Can you work these out from the model? Positions are in its coordinate system, mm. Face numbers are marked on the shaded views. A direction names the side the tool comes from. Coordinates: 2 decimals unless noted, no trailing zeros. Write each loop counter-clockwise with the first axis right and the second up, starting at its lowest first coordinate (ties: lowest second). Pieces come first, ordered by that corner, then holes. Notation, with made-up numbers: (39, 14) -> (63, 14) arc R25 cw to (63, 32) -> close; hole circle Ø3 at (84, 14). An arc over 180 degrees is marked (long way). Use one line per item in the form item = value.
```python
from build123d import *

# Parameters (mm, degrees)
F0_W     = 16
F0_H     = 16
F1_DEPTH = 220
F2_R     = 7.99999
F3_R     = 7.5
F4_DEPTH = 20


# Not quite as in the source:
# - a fillet or chamfer is up to 0.001 mm smaller than in the source, because OpenCascade refuses the exact size


with BuildPart() as f1:
    # F0 (on Top) → F1 (new body)
    with BuildSketch(Plane.XY):
        with Locations((-0.2842125371, -4.0679279789)):
            Rectangle(F0_W, F0_H)
    extrude(amount=F1_DEPTH)

    # F2 (radius 8 in the source; OpenCascade refuses exactly that, so slightly less here)
    f2_edges = [f1.edges().sort_by_distance(p)[0] for p in [
        (-8.284213, -12.067928, 110),
        (7.715787, -12.067928, 110),
    ]]
    fillet(f2_edges, radius=F2_R)

    # F3 (on face) → F4 (join)
    with BuildSketch(Plane(origin=(0, 3.9320720211, 0), x_dir=(-1, 0, 0), z_dir=(0, 1, 0))):
        with Locations((0.2842125371, 185.9523057938)):
            Circle(F3_R)
    extrude(amount=F4_DEPTH)


solid = f1.part
```
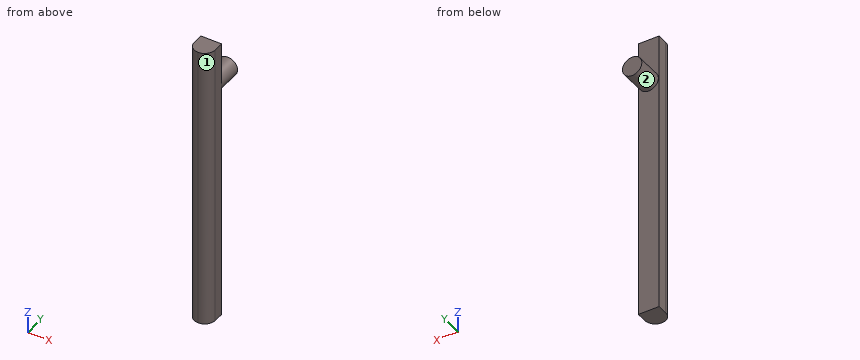
Q1. If I drill on line 1 (Y direction, x = 0.5, z = 90.5); line 2 (Z direction, x = 0, y = 9); line 3 (Y direction, x = -1, z = 189), over which ranges is the centre line in solid material (lowest first)? Write a range as from..to.
Return value:
line_1 = -12.03..3.93
line_2 = 178.46..193.45
line_3 = -12.04..23.93
Q2. Suppose I cut it at C-C (y = -7.5). Write out the boundary of the cut face in (x, z).
Return value:
outline = (-7.51, 0) -> (6.94, 0) -> (6.94, 220) -> (-7.51, 220) -> close
Q3. Suppose I cut it at B-B (x = 4.25). Write out the boundary of the cut face in (y, z).
Return value:
outline = (-10.66, 0) -> (3.93, 0) -> (3.93, 179.98) -> (23.93, 179.98) -> (23.93, 191.93) -> (3.93, 191.93) -> (3.93, 220) -> (-10.66, 220) -> close
Q4. Will these pins go through, and if not, where does the flat tip stop? pin 1 (12 mm diameter, centred on y = -8.5, z = 188.5, fed in from -X); pin 2 (8 mm diameter, centred on x = -2, y = 8.5, fed in from +Z); pin 3 (4 mm diameter, centred on x = -5.5, z = 100.5, fed in from -Y).
Return value:
pin_1 = -8.28
pin_2 = 193.45
pin_3 = -11.39
Q5. For the marked faces 1 and 2, which set-ups out of +Z, -Z, +X, -X, +Y, -Y let a thin tool reach every point of the face, with its end or its side?
Return value:
face_1 = +Z, -Z, +X, -Y
face_2 = +Y
Q6. Suppose I cut it at D-D (x = -4.5). Write out the boundary of the cut face in (y, z).
Return value:
outline = (-10.87, 0) -> (3.93, 0) -> (3.93, 179.75) -> (23.93, 179.75) -> (23.93, 192.16) -> (3.93, 192.16) -> (3.93, 220) -> (-10.87, 220) -> close
